from build123d import *

# Parameters (mm, degrees)
SKETCH1_W                      = 488.95
SKETCH1_H                      = 128
BOSS_EXTRUDE1_DEPTH            = 5
CBORE_FOR_M4_SHCS1_D           = 4.5
CBORE_FOR_M4_SHCS1_DEPTH       = 17.38
CBORE_FOR_M4_SHCS1_CBORE_D     = 8
CBORE_FOR_M4_SHCS1_CBORE_DEPTH = 4
CBORE_FOR_M4_SHCS1_TIP         = 1.351936393
FILLET1_R                      = 2.5
CUT_EXTRUDE1_DEPTH             = 253.762785285
LPATTERN1_COUNT                = 5
LPATTERN1_PITCH                = 96


with BuildPart() as part:
    # Sketch1 → Boss-Extrude1 (new body)
    with BuildSketch(Plane(origin=(0, 0, 0), x_dir=(1, 0, 0), z_dir=(0, 1, 0))):
        Rectangle(SKETCH1_W, SKETCH1_H)
    extrude(amount=BOSS_EXTRUDE1_DEPTH)

    # CBORE for M4 SHCS1
    with Locations(Plane(origin=(0, 5, 0), x_dir=(1, 0, 0), z_dir=(0, 1, 0))):
        with Locations((-239.475, 59), (-239.475, -59), (239.475, -59), (239.475, 59)):
            CounterBoreHole(CBORE_FOR_M4_SHCS1_D / 2, CBORE_FOR_M4_SHCS1_CBORE_D / 2, CBORE_FOR_M4_SHCS1_CBORE_DEPTH, depth=CBORE_FOR_M4_SHCS1_DEPTH)
            with Locations((0, 0, -(CBORE_FOR_M4_SHCS1_DEPTH + CBORE_FOR_M4_SHCS1_TIP / 2))):  # 118° drill point
                Cone(0, CBORE_FOR_M4_SHCS1_D / 2, CBORE_FOR_M4_SHCS1_TIP, mode=Mode.SUBTRACT)

    # Fillet1
    fillet1_edges = [part.edges().sort_by_distance(p)[0] for p in [
        (244.475, 2.5, 64),
        (-244.475, 2.5, 64),
        (-244.475, 2.5, -64),
        (244.475, 2.5, -64),
    ]]
    fillet(fillet1_edges, radius=FILLET1_R)

    # Sketch4 → Cut-Extrude1 (cut, through all)
    with BuildSketch(Plane(origin=(0, 5, 0), x_dir=(1, 0, 0), z_dir=(0, 1, 0))):
        with BuildLine():
            Line((-196.975, 20.25), (-186.975, 20.25))
            ThreePointArc((-186.975, 20.25), (-184.725, 18), (-186.975, 15.75))
            Line((-186.975, 15.75), (-196.975, 15.75))
            ThreePointArc((-196.975, 15.75), (-199.225, 18), (-196.975, 20.25))
        make_face()
        with BuildLine():
            Line((-196.975, -15.75), (-186.975, -15.75))
            ThreePointArc((-186.975, -15.75), (-184.725, -18), (-186.975, -20.25))
            Line((-186.975, -20.25), (-196.975, -20.25))
            ThreePointArc((-196.975, -20.25), (-199.225, -18), (-196.975, -15.75))
        make_face()
    cut_extrude1 = extrude(amount=-CUT_EXTRUDE1_DEPTH, mode=Mode.SUBTRACT)

    # LPattern1: Cut-Extrude1 ×5
    with Locations(*[(i * LPATTERN1_PITCH, 0, 0) for i in range(1, LPATTERN1_COUNT)]):
        add(cut_extrude1, mode=Mode.SUBTRACT)


solid = part.part
For this review, take the finished solid that the model builds, in its own axes (mm). A direction names the side the tool comes from. Round coordinates to 2 decimals unless told otherwise and drop trailing zeros. Use a Markdown table: item, result. Add a question column.
Item 1: Tool access review of faces 3 (the flat face through (-3, 5, -1)), 4 (the cylindrical face through (236.3, 3.03, -56.57)): name each direction out of +Z, -Z, +X, -X, +Y, -Y from which nothing blocks a thin tool from reaching the whole face with its end or side.
Item 2: To check wall thickness, follow line 1 along Z through (x, y) = (-192, 3.95); line 2 along X through (y, z) = (3.75, -59) (3 decimals); line 3 along X through (y, z) = (4.2, 17) (3 decimals). State the ranges of each line that lie inside material, in increasing order.
Item 3: Mouldability with a two-part tool opening along Z and no side actions: class faces 1 (the flat face through (-3, 0, -1)), 2 (the cylindrical face through (-235.78, 3.03, -57.47)) as released by +Z, released by -Z, zero draft, split by the parting line, or undercut.
Item 4: Insertion check: pin 1 (7 mm diameter, centred on x = -239.475, z = 59, fed in from +Y). The pin has a flat end and moves straight along its axis. Give the tip position at first contact, or say it passes through.
Geometry results:
| question | item | result |
|---|---|---|
| 1 | face 3 | +Z, -Z, +X, -X, +Y |
| 1 | face 4 | +Y |
| 2 | line 1 | z = -64 to -20.25, -15.75 to 15.75, 20.25 to 64 |
| 2 | line 2 | x = -244.475 to -243.475, -235.475 to 235.475, 243.475 to 244.475 |
| 2 | line 3 | x = -244.475 to -198.991, -184.959 to -102.991, -88.959 to -6.991, 7.041 to 89.009, 103.041 to 185.009, 199.041 to 244.475 |
| 3 | face 1 | zero draft |
| 3 | face 2 | undercut |
| 4 | pin 1 | stops at y = 1 |
